Design review of the part built by this model. Coordinates are the model's own, in mm. A direction names the side the tool comes from. Coordinates: 2 decimals unless noted, no trailing zeros. Write each loop counter-clockwise with the first axis right and the second up, starting at its lowest first coordinate (ties: lowest second). Pieces come first, ordered by that corner, then holes. Notation, with made-up numbers: (56.25, 25.25) -> (107.25, 25.25) arc R18 ccw to (107.25, 50.25) -> close; hole circle Ø8 at (38.5, -5). An arc over 180 degrees is marked (long way). Return JSON: item names as keys, results as strings. Group by question number.
from build123d import *

# Parameters (mm, degrees)
F0_R      = 50
F1_DEPTH  = 75
F2_R      = 25
F3_DEPTH  = 50
F4_R      = 20
F5_DEPTH  = 10
F6_R      = 25
F7_DEPTH  = 35
F8_R      = 20
F9_DEPTH  = 10
F10_R     = 25
F11_DEPTH = 40
F12_R     = 20
F13_DEPTH = 10
F14_R     = 25
F15_DEPTH = 40
F17_DEPTH = 25
F19_ANGLE = 90
F22_R     = 25
F23_DEPTH = 50


# Not quite as in the source:
# - a feature names something its author has since deleted; it is built from what else it names


with BuildPart() as f1:
    # F0 (on Front) → F1 (new body)
    with BuildSketch(Plane.XZ):
        Circle(F0_R)
    extrude(amount=F1_DEPTH)

    # F2 (on face) → F3 (join)
    with BuildSketch(Plane(origin=(0, 0, 0), x_dir=(-1, 0, 0), z_dir=(0, 1, 0))):
        Circle(F2_R)
    extrude(amount=F3_DEPTH)

    # F4 (on face) → F5 (join)
    with BuildSketch(Plane(origin=(0, 50, 0), x_dir=(-1, 0, 0), z_dir=(0, 1, 0))):
        Circle(F4_R)
    extrude(amount=F5_DEPTH)

    # F6 (on face) → F7 (join)
    with BuildSketch(Plane(origin=(0, 60, 0), x_dir=(-1, 0, 0), z_dir=(0, 1, 0))):
        Circle(F6_R)
    extrude(amount=F7_DEPTH)

    # F8 (on face) → F9 (join)
    with BuildSketch(Plane(origin=(0, 95, 0), x_dir=(-1, 0, 0), z_dir=(0, 1, 0))):
        Circle(F8_R)
    extrude(amount=F9_DEPTH)

    # F10 (on face) → F11 (join)
    with BuildSketch(Plane(origin=(0, 105, 0), x_dir=(-1, 0, 0), z_dir=(0, 1, 0))):
        Circle(F10_R)
    extrude(amount=F11_DEPTH)

    # F12 (on face) → F13 (join)
    with BuildSketch(Plane(origin=(0, 145, 0), x_dir=(-1, 0, 0), z_dir=(0, 1, 0))):
        Circle(F12_R)
    extrude(amount=F13_DEPTH)

    # F14 (on face) → F15 (join)
    with BuildSketch(Plane(origin=(0, 155, 0), x_dir=(-1, 0, 0), z_dir=(0, 1, 0))):
        Circle(F14_R)
    extrude(amount=F15_DEPTH)

    # F16 (on face) → F17 (join)
    with BuildSketch(Plane(origin=(0, 195, 0), x_dir=(-1, 0, 0), z_dir=(0, 1, 0))):
        Polygon((12.5, 21.6506350946), (-12.5, 21.6506350946), (-25, 0), (-12.5, -21.6506350946), (12.5, -21.6506350946), (25, 0), align=None)
    extrude(amount=F17_DEPTH)

    # F18 (on face) → F19 (revolve, cut)
    with BuildSketch(Plane.XZ.offset(75)):
        with BuildLine():
            ThreePointArc((50, 0), (41.8330013267, 27.3861278753), (20, 45.8257569496))
            Line((20, 45.8257569496), (20, -45.8257569496))
            ThreePointArc((20, -45.8257569496), (41.8330013267, -27.3861278753), (50, 0))
        make_face()
    revolve(axis=Axis((70, -75, -0.5619522762), (0, 0, -1)), revolution_arc=F19_ANGLE, mode=Mode.SUBTRACT)

    # F20 (on face) → F21 (revolve, cut)
    with BuildSketch(Plane.XZ.offset(75)):
        with BuildLine():
            Line((-20, -45.8257569496), (-20, 45.8257569496))
            ThreePointArc((-20, 45.8257569496), (-50, 0), (-20, -45.8257569496))
        make_face()
    revolve(axis=Axis((-70, -75, -0.6762938916), (0, 0, -1)), mode=Mode.SUBTRACT)

    # F22 (on Right) → F23 (cut, symmetric)
    with BuildSketch(Plane.YZ):
        with Locations((-75, 0)):
            Circle(F22_R)
    extrude(amount=F23_DEPTH, both=True, mode=Mode.SUBTRACT)


solid = f1.part
Q1. Wall thickness on L1, parallel to Y at x = -7, z = -35; L2, parallel to Z at x = -0.5, y = -10; L3, parallel to Y at x = 8, z = 0: over which ranges is each line inside the solid? List them lowest first.
Q2. We need section B-B on y = 27. Write out the cut boundary in (x, z), plus the area to 3 significant figures.
Q3. We need section A-A on z = 28. Write out the cut boundary in (x, y), plus the area to 3 significant figures.
Q4. For faces 5 (the flat face through (-18.84, 207.32, 10.67)), 6 (the cylindrical face through (4.336, 149.93, -19.524)), 7 (the cylindrical face through (-23.846, 77.255, 7.509)), 8 (the flat face through (20, 195, -12)), list the 3-axis set-ups (+Z, -Z, +X, -X, +Y, -Y) from which the entire face can be reached by the end or side of a thin tool; tool diameter is ignored.
Q5. The part is to be moulded in two halves that separate along Y. For faces 1 (the flat face through (11, 50, 17)), 2 (the cylindrical face through (-23.846, 174.72, 7.509)), 3 (the flat face through (0, 220, 0)), 4 (the cylindrical face through (4.336, 99.93, -19.524)), say which applies: +Y half, -Y half, draft (parallel to the pull), parting line (faces both ways), or undercut.
Q6. For P1, Ø1.5, axis at y = -44, z = 30.5, coming from the +X side; P2, Ø10, axis at x = -7.5, z = 32.5, coming from the +Y side; P3, Ø12.5, axis at x = -1, y = 202, coming from the -Z side; P4, Ø4, axis at x = -17, z = -16, coming from the +Y side, all flat-tipped, find the tip position at first contact; note any pin that passes through.
Q7. We need section C-C on x = 40. Write out the cut boundary in (y, z).
Findings below:
{
 "1": {"L1": "y = -75 to 0", "L2": "z = -50 to 50", "L3": "y = -50 to 220"},
 "2": {"outline": "circle Ø50 at (0, 0)", "area": "1,960 mm^2"},
 "3": {"outline": "(-41.42, -33.97) arc R50 cw to (-20, -75) -> (20, -75) arc R50 cw to (41.42, -33.97) -> (41.42, 0) -> (-41.42, 0) -> close", "area": "4,980 mm^2"},
 "4": {"face 5": "+Z, -X, +Y", "face 6": "none", "face 7": "+Y", "face 8": "-Z, +X, +Y"},
 "5": {"face 1": "undercut", "face 2": "draft", "face 3": "+Y half", "face 4": "undercut"},
 "6": {"P1": "stops at x = 31.37", "P2": "stops at y = 0", "P3": "stops at z = -21.65", "P4": "stops at y = 220"},
 "7": {"outline": "(-35, -30) -> (0, -30) -> (0, 30) -> (-35, 30) -> close"}
}
